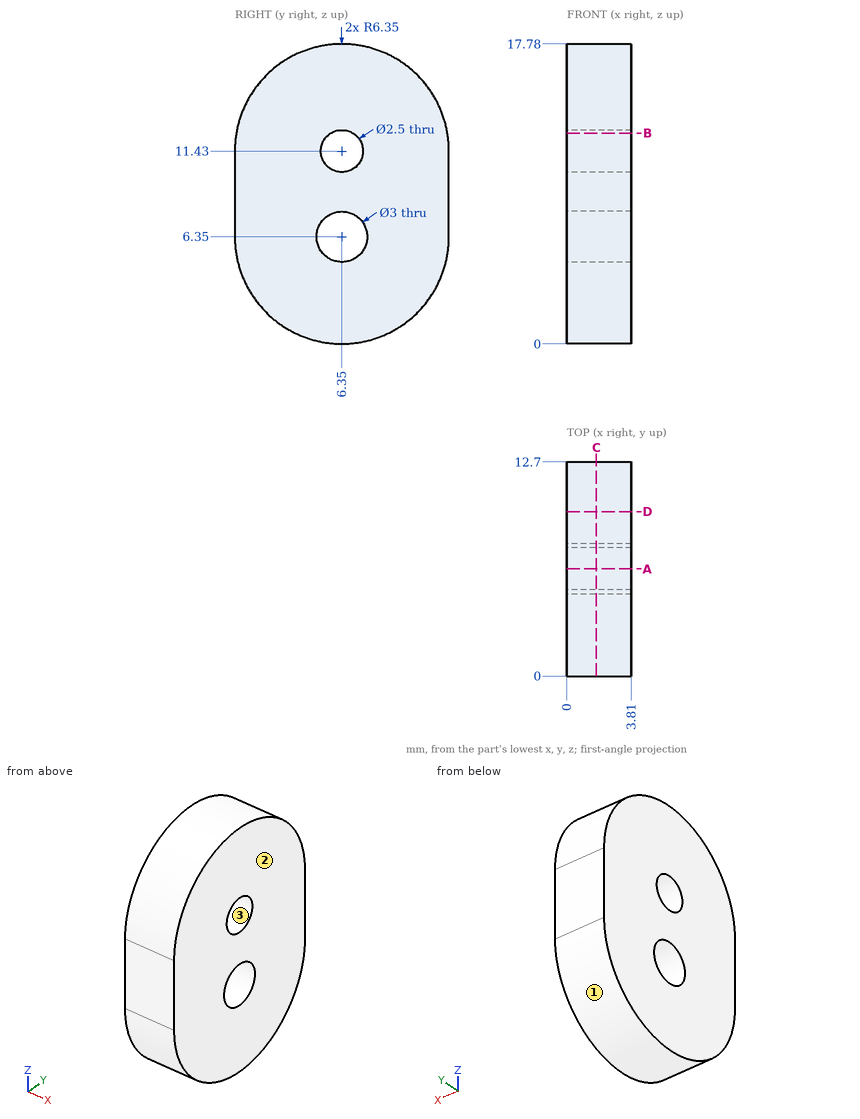
Part print with two shaded views. Sizes in mm from the minimum x, y, z corner. Round coordinates to 2 decimals unless told otherwise and drop trailing zeros. Write each loop counter-clockwise with the first axis right and the second up, starting at its lowest first coordinate (ties: lowest second). Pieces come first, ordered by that corner, then holes. Notation, with made-up numbers: M -22,19 L 9,19 A19 cw 9,42 Z; hole C 32.25,87 d4. An arc over 180 degrees is marked long. Answer as CSV lines item,"result". Start each with the question number.
1) Mould opens along Z. For the marked faces 1, 2 and 3 say: +Z half, -Z half, draft (parallel to the pull), parting line (faces both ways), or undercut.
2) Band-saw the part on D-D (y = 9.75). List the corners of the cut face in (x, z).
3) Band-saw the part on C-C (x = 1.75). List the corners of the cut face in (y, z), then the cut area to 3 significant figures.
4) Drill centre lines: L1, parallel to Z at x = 0.9, y = 6.25; L2, parallel to Y at x = 1.65, z = 11.43; L3, parallel to Y at x = 2.05, z = 6.35. Where is each one in solid material? Low to high.
5) Band-saw the part on A-A (y = 6.35). List the corners of the cut face in (x, z).
6) Band-saw the part on B-B (z = 12.5). List the corners of the cut face in (x, y), then the cut area to 3 significant figures.
7) Drop flat-ended pins along their axis: pin 1 (1.5 mm diameter, centred on x = 0.5, z = 12.5, fed in from +Y); pin 2 (1.5 mm diameter, centred on x = 3, z = 13, fed in from -Y); pin 3 (1 mm diameter, centred on x = 0.5, z = 13.5, fed in from +Y). Give the stop position or say it passes through.
Worked out:
1,face 1,"-Z half"
1,face 2,"draft"
1,face 3,"undercut"
2,outline,"M 0,0.99 L 3.81,0.99 L 3.81,16.79 L 0,16.79 Z"
3,outline,"M 0,6.35 A6.35 ccw 12.7,6.35 L 12.7,11.43 A6.35 ccw 0,11.43 Z; hole C 6.35,6.35 d3; hole C 6.35,11.43 d2.5"
3,area,"179 mm²"
4,L1,"0 to 4.85, 7.85 to 10.18, 12.68 to 17.78"
4,L2,"0 to 5.1, 7.6 to 12.7"
4,L3,"0 to 4.85, 7.85 to 12.7"
5,outline,"M 0,0 L 3.81,0 L 3.81,4.85 L 0,4.85 Z; M 0,7.85 L 3.81,7.85 L 3.81,10.18 L 0,10.18 Z; M 0,12.68 L 3.81,12.68 L 3.81,17.78 L 0,17.78 Z"
6,outline,"M 0,0.09 L 3.81,0.09 L 3.81,5.7 L 0,5.7 Z; M 0,7 L 3.81,7 L 3.81,12.61 L 0,12.61 Z"
6,area,"42.8 mm²"
7,pin 1,"y = 12.69"
7,pin 2,"y = 0.05"
7,pin 3,"y = 12.5"
